Geometry: see drawing. Coordinates: mm, zero at the bounding-box minimum. Coordinates: 2 decimals unless noted, no trailing zeros. Write each loop counter-clockwise with the first axis right and the second up, starting at its lowest first coordinate (ties: lowest second). Pieces come first, ordered by that corner, then holes. Notation, with made-up numbers: M 22.5,-13.5 L 49.5,-13.5 A28 ccw 49.5,8.5 Z; hole C 52,11.25 d4. An arc over 180 degrees is marked long. One line per item, written item: value. Start each with the question number.
Item 1: Cut plane B-B, the plane x = 20.25. Output: boundary loops of the cut face in (y, z), then the cut area to 3 significant figures.
Item 2: Mould query, pull axis X, two halves, no side actions, for the marked faces 1, 2 and 3. Classes: released by +X, released by -X, zero draft, split by the parting line, or undercut.
Item 3: Ray query, L1, parallel to X at y = 11.25, z = 25; L2, parallel to Y at x = 18.95, z = 20; L3, parallel to Y at x = 14.5, z = 26.5. Return the intervals inside material, ascending. Write a range as from..to.
Item 4: Pin query (flat end, axial travel): P1, Ø2, axis at x = 13.5, y = 20, coming from the -Z side; P2, Ø1.5, axis at x = 8.5, y = 10.5, coming from the +Z side; P3, Ø4, axis at x = 17.5, z = 34, coming from the +Y side. Return the tip coordinate at first contact, or that it passes through.
Item 5: Cut plane C-C, the plane y = 21. Output: boundary loops of the cut face in (x, z).
Item 6: Cut plane D-D, the plane y = 14.25. Output: boundary loops of the cut face in (x, z).
Item 7: Cut plane A-A, the plane z = 20. Output: boundary loops of the cut face in (x, y), then the cut area to 3 significant figures.
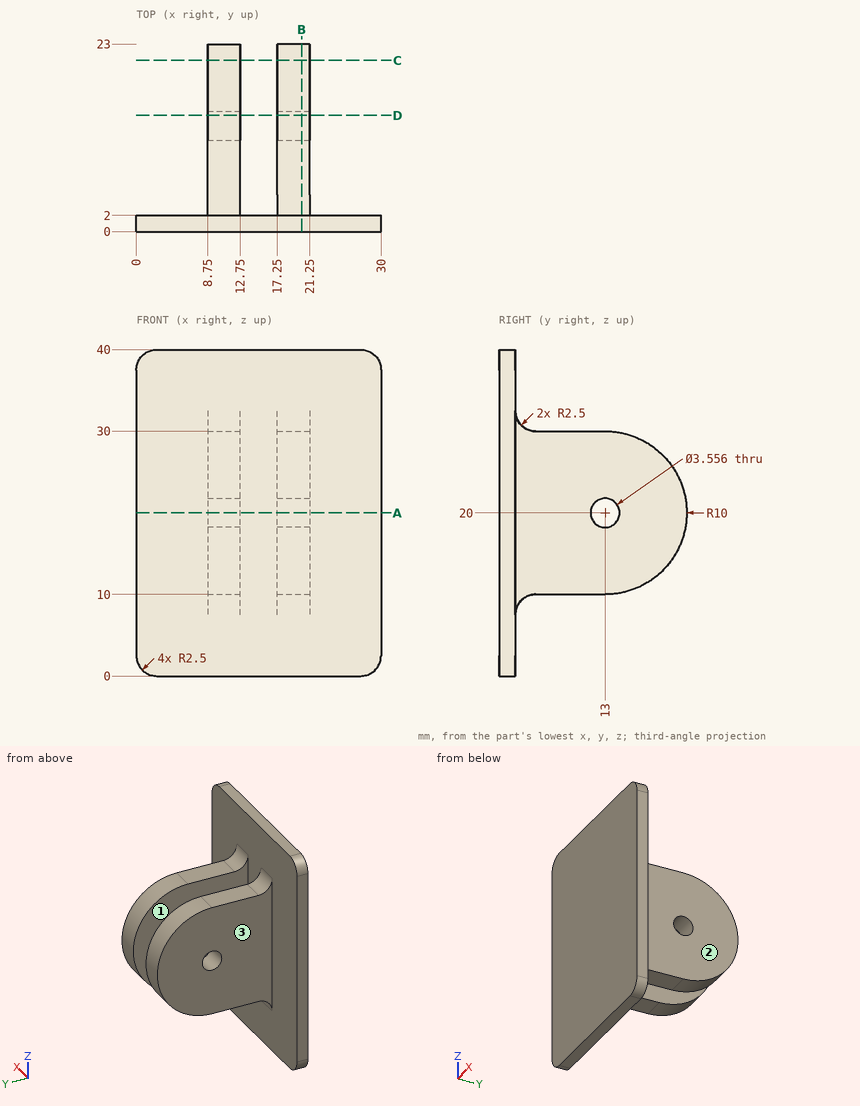
From the geometry:
1. outline: M 0,0 L 2,0 L 2,7.5 A2.5 cw 4.5,10 L 13,10 A10 ccw 13,30 L 4.5,30 A2.5 cw 2,32.5 L 2,40 L 0,40 Z; hole C 13,20 d3.56
1. area: 450 mm²
2. face 1: undercut
2. face 2: released by +X
2. face 3: released by -X
3. L1: x = 8.75..12.75, 17.25..21.25
3. L2: y = 0..11.22, 14.78..23
3. L3: y = 0..2
4. P1: stops at z = 12.27
4. P2: stops at z = 30
4. P3: stops at y = 2.05
5. outline: M 8.75,14 L 12.75,14 L 12.75,26 L 8.75,26 Z; M 17.25,14 L 21.25,14 L 21.25,26 L 17.25,26 Z
6. outline: M 8.75,10.08 L 12.75,10.08 L 12.75,18.74 L 8.75,18.74 Z; M 8.75,21.26 L 12.75,21.26 L 12.75,29.92 L 8.75,29.92 Z; M 17.25,10.08 L 21.25,10.08 L 21.25,18.74 L 17.25,18.74 Z; M 17.25,21.26 L 21.25,21.26 L 21.25,29.92 L 17.25,29.92 Z
7. outline: M 0,0 L 30,0 L 30,2 L 21.25,2 L 21.25,11.22 L 17.25,11.22 L 17.25,2 L 12.75,2 L 12.75,11.22 L 8.75,11.22 L 8.75,2 L 0,2 Z; M 8.75,14.78 L 12.75,14.78 L 12.75,23 L 8.75,23 Z; M 17.25,14.78 L 21.25,14.78 L 21.25,23 L 17.25,23 Z
7. area: 200 mm²
